```python
from build123d import *

# Parameters (mm, degrees)
SKETCH_1_W      = 16
SKETCH_1_H      = 40
SKETCH_1_R      = 2.5
SKETCH_1_R_2    = 5
EXTRUDE_1_DEPTH = 5
FILLET_1_R      = 3


with BuildPart() as part:
    # 草图1 → 凸台-拉伸1 (new body)
    with BuildSketch(Plane.XY):
        with Locations((0, 12.5)):
            Rectangle(SKETCH_1_W, SKETCH_1_H)
        with Locations((0, 25)):
            Circle(SKETCH_1_R, mode=Mode.SUBTRACT)
        Circle(SKETCH_1_R, mode=Mode.SUBTRACT)
        with Locations((0, 12.5)):
            Circle(SKETCH_1_R_2, mode=Mode.SUBTRACT)
    extrude(amount=EXTRUDE_1_DEPTH)

    # 圆角1
    fillet_1_edges = [part.edges().sort_by_distance(p)[0] for p in [
        (8, -7.5, 2.5),
        (-8, -7.5, 2.5),
        (-8, 32.5, 2.5),
        (8, 32.5, 2.5),
    ]]
    fillet(fillet_1_edges, radius=FILLET_1_R)


solid = part.part
```
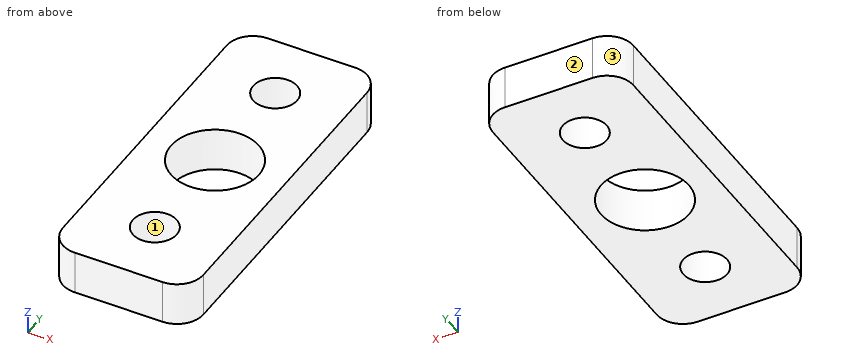
Check sheet for the modelled part. Datum: model origin and axes. Units: mm. Face numbers are marked on the shaded views. Round coordinates to 2 decimals unless told otherwise and drop trailing zeros. Loops run counter-clockwise (first coordinate to the right, second up) from the corner with the lowest first, then second, coordinate; pieces in that order, holes last. Notation, with made-up numbers: (41, 77) - (100, 77) arc R24 cw to (100, 114) - close; hole circle Ø1 at (-18.5, -3). An arc over 180 degrees is marked (long way). Answer as a JSON object with one key per item and string values. Group by question number.
Q1. Sectioned sample at D-D, the plane x = 1.5. Enter the section's corners in (y, z), plus the area to 3 significant figures.
Q2. Scan lines: line 1 along Y through (x, z) = (0, 2.65); line 2 along Y through (x, z) = (-0.5, 3.85); line 3 along X through (y, z) = (26.5, 1.85). Record each from-to range of solid material in increasing order. Write a range as [from, to].
Q3. Sectioned sample at A-A, the plane y = 0. Enter the section's corners in (x, z).
Q4. Sectioned sample at C-C, the plane x = 4.25. Enter the section's corners in (y, z).
Q5. Sectioned sample at B-B, the plane z = 3.35. Enter the section's corners in (x, y), plus the area to 3 significant figures.
Q6. Mould release check, pull along X, two halves, no side actions. Record for the marked faces 1, 2 and 3: released by +X, released by -X, zero draft, split by the parting line, or undercut.
Solution:
{
 "1": {"outline": "(-7.5, 0) - (-2, 0) - (-2, 5) - (-7.5, 5) - close; (2, 0) - (7.73, 0) - (7.73, 5) - (2, 5) - close; (17.27, 0) - (23, 0) - (23, 5) - (17.27, 5) - close; (27, 0) - (32.5, 0) - (32.5, 5) - (27, 5) - close", "area": "112 mm²"},
 "2": {"line 1": "y = [-7.5, -2.5], [2.5, 7.5], [17.5, 22.5], [27.5, 32.5]", "line 2": "y = [-7.5, -2.45], [2.45, 7.53], [17.47, 22.55], [27.45, 32.5]", "line 3": "x = [-8, -2], [2, 8]"},
 "3": {"outline": "(-8, 0) - (-2.5, 0) - (-2.5, 5) - (-8, 5) - close; (2.5, 0) - (8, 0) - (8, 5) - (2.5, 5) - close"},
 "4": {"outline": "(-7.5, 0) - (9.87, 0) - (9.87, 5) - (-7.5, 5) - close; (15.13, 0) - (32.5, 0) - (32.5, 5) - (15.13, 5) - close"},
 "5": {"outline": "(-8, -4.5) arc R3 ccw to (-5, -7.5) - (5, -7.5) arc R3 ccw to (8, -4.5) - (8, 29.5) arc R3 ccw to (5, 32.5) - (-5, 32.5) arc R3 ccw to (-8, 29.5) - close; hole circle Ø10 at (0, 12.5); hole circle Ø5 at (0, 0); hole circle Ø5 at (0, 25)", "area": "514 mm²"},
 "6": {"face 1": "undercut", "face 2": "zero draft", "face 3": "released by -X"}
}
